from build123d import *

# Parameters (mm, degrees)
SKETCH1_W             = 40
SKETCH1_H             = 44.999999916
VERTICAL_BASE_DEPTH   = 1
TOP_ROUNDING_R        = 20
TOP_ROUNDING_2_R      = 20
SKETCH2_W             = 40
SKETCH2_H             = 1
HORIZONTAL_BASE_DEPTH = 41
FILLET3_R             = 2.54
FILLET4_R             = 2.54
SKETCH3_R             = 1.75
MOUNTING_HOLES_DEPTH  = 73.801098842
SKETCH5_W             = 13
SKETCH5_H             = 27
CUT_EXTRUDE2_DEPTH    = 74.409808557
FILLET5_R             = 6.5
FILLET6_R             = 6.5
FILLET7_R             = 6.5
FILLET8_R             = 6.5


with BuildPart() as part:
    # Sketch1 → Vertical-Base (new body)
    with BuildSketch(Plane.XY):
        with Locations((20, 22.499999958)):
            Rectangle(SKETCH1_W, SKETCH1_H)
    extrude(amount=VERTICAL_BASE_DEPTH)

    # Top-Rounding
    top_rounding_edges = [part.edges().sort_by_distance(p)[0] for p in [
        (0, 44.999999916, 0.5),
    ]]
    fillet(top_rounding_edges, radius=TOP_ROUNDING_R)

    # Top-Rounding-2
    top_rounding_2_edges = [part.edges().sort_by_distance(p)[0] for p in [
        (40, 44.999999916, 0.5),
    ]]
    fillet(top_rounding_2_edges, radius=TOP_ROUNDING_2_R - 0.0001)  # a hair under: the kernel refuses the full size

    # Sketch2 → Horizontal-Base (add)
    with BuildSketch(Plane.XY.offset(1)):
        with Locations((20, 0.5)):
            Rectangle(SKETCH2_W, SKETCH2_H)
    extrude(amount=HORIZONTAL_BASE_DEPTH)

    # Fillet3
    fillet3_edges = [part.edges().sort_by_distance(p)[0] for p in [
        (40, 0.5, 42),
    ]]
    fillet(fillet3_edges, radius=FILLET3_R)

    # Fillet4
    fillet4_edges = [part.edges().sort_by_distance(p)[0] for p in [
        (0, 0.5, 42),
    ]]
    fillet(fillet4_edges, radius=FILLET4_R)

    # Sketch3 → Mounting Holes (cut, through all)
    with BuildSketch(Plane(origin=(0, 1, 0), x_dir=(1, 0, 0), z_dir=(0, 1, 0))):
        with Locations(Location((35, -32.979707006, 0), (0, 0, 270))):
            Circle(SKETCH3_R)
        with Locations(Location((5, -32.979707006, 0), (0, 0, 270))):
            Circle(SKETCH3_R)
        with Locations(Location((5, -9.020292994, 0), (0, 0, 270))):
            Circle(SKETCH3_R)
        with Locations(Location((35, -9.020292994, 0), (0, 0, 270))):
            Circle(SKETCH3_R)
    extrude(amount=-MOUNTING_HOLES_DEPTH, mode=Mode.SUBTRACT)

    # Sketch5 → Cut-Extrude2 (cut, through all)
    with BuildSketch(Plane(origin=(0, 0, 0), x_dir=(-1, 0, 0), z_dir=(0, 0, -1))):
        with Locations((-20, 27)):
            Rectangle(SKETCH5_W, SKETCH5_H)
    extrude(amount=-CUT_EXTRUDE2_DEPTH, mode=Mode.SUBTRACT)

    # Fillet5
    fillet5_edges = [part.edges().sort_by_distance(p)[0] for p in [
        (13.5, 40.5, 0.5),
    ]]
    fillet(fillet5_edges, radius=FILLET5_R)

    # Fillet6
    fillet6_edges = [part.edges().sort_by_distance(p)[0] for p in [
        (26.5, 40.5, 0.5),
    ]]
    fillet(fillet6_edges, radius=FILLET6_R - 0.0001)  # a hair under: the kernel refuses the full size

    # Fillet7
    fillet7_edges = [part.edges().sort_by_distance(p)[0] for p in [
        (13.5, 13.5, 0.5),
    ]]
    fillet(fillet7_edges, radius=FILLET7_R)

    # Fillet8
    fillet8_edges = [part.edges().sort_by_distance(p)[0] for p in [
        (26.5, 13.5, 0.5),
    ]]
    fillet(fillet8_edges, radius=FILLET8_R - 0.0001)  # a hair under: the kernel refuses the full size


solid = part.part
Work out the finished part from the listing and answer in its coordinate system (mm). A direction names the side the tool comes from. Give positions to 0.01 mm unless a question says otherwise; leave off trailing zeros. Loops run counter-clockwise (first coordinate to the right, second up) from the corner with the lowest first, then second, coordinate; pieces in that order, holes last. Notation, with made-up numbers: M 1.25,82 L 9.25,82 A23 cw 9.25,97 Z; hole C 33,-26 d6. An arc over 180 degrees is marked long. Use CSV: the item, a comma, the result in double quotes.
1) Find section C-C on z = 34. Write down the section's boundary in (x, y), plus the area to 3 significant figures.
Answer:
outline,"M 0,0 L 3.58,0 L 3.58,1 L 0,1 Z; M 6.42,0 L 33.58,0 L 33.58,1 L 6.42,1 Z; M 36.42,0 L 40,0 L 40,1 L 36.42,1 Z"
area,"34.3 mm^2"
2) Given P1, Ø4.5, axis at x = 35, z = 32.98, coming from the +Y side; P2, Ø1.1, axis at y = 27.5, z = 0.5, coming from the +X side, each flat-ended and moving along its own axis, determine where each tip first touches the part or whether it passes through.
Answer:
P1,"y = 1"
P2,"x = 39.9"
3) Find section B-B on y = 27. Write down the section's boundary in (x, z).
Answer:
outline,"M 0.1,0 L 13.5,0 L 13.5,1 L 0.1,1 Z; M 26.5,0 L 39.9,0 L 39.9,1 L 26.5,1 Z"
4) Determine the mould class of faces 1 (the flat face through (24, 14, 1)), 2 (the cylindrical face through (4.33, 0.507, 34.596)), 3 (the flat face through (40, 0.4, 10.9)), 4 (the cylindrical face through (15.354, 15.455, 0.507)) for opening direction X: released by +X, released by -X, zero draft, split by the parting line, or undercut.
Answer:
face 1,"zero draft"
face 2,"undercut"
face 3,"released by +X"
face 4,"undercut"
5) Find section A-A on x = 35. Write down the section's boundary in (y, z).
Answer:
outline,"M 0,0 L 38.23,0 L 38.23,1 L 1,1 L 1,7.27 L 0,7.27 Z; M 0,10.77 L 1,10.77 L 1,31.23 L 0,31.23 Z; M 0,34.73 L 1,34.73 L 1,42 L 0,42 Z"
6) Which of the six approach directions +Z, -Z, +X, -X, +Y, -Y give full straight-line access (tool end or side, diameter ignored) to faces 5 (the flat face through (20, 1, 21)), 6 (the cylindrical face through (24.545, 38.646, 0.507)), 7 (the cylindrical face through (39.276, 0.507, 41.236))?
Answer:
face 5,"+Z, +X, -X, +Y"
face 6,"+Z, -Z"
face 7,"+Z, +X, +Y, -Y"
7) Consider L1, parallel to Y at x = 7, z = 35.5. Determine where the line is inside the solid, lowest interval first.
Answer:
L1,"0 to 1"
8) Find section D-D on x = 18. Write down the section's boundary in (y, z).
Answer:
outline,"M 0,0 L 13.82,0 L 13.82,1 L 1,1 L 1,42 L 0,42 Z; M 40.18,0 L 44.9,0 L 44.9,1 L 40.18,1 Z"
